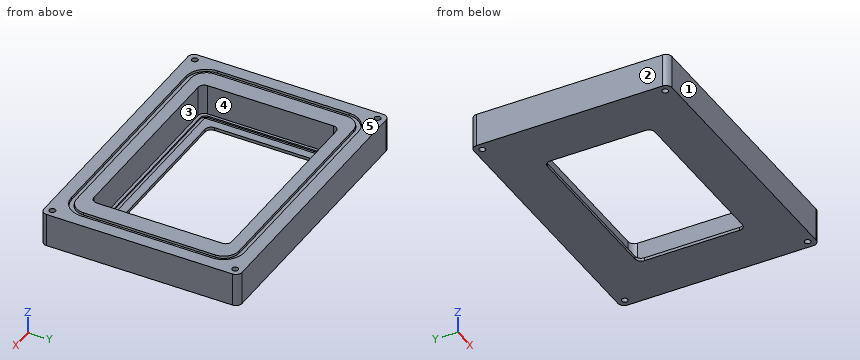
Autodesk Fusion 360 part; units mm, degrees
sketch "Sketch1" plane through (0, 0, 0) normal (0, 0, 1) x (1, 0, 0)
  line L0 (86, -65) -> (-86, -65)
  line L1 (-90, -61) -> (-90, 61)
  line L2 (-86, 65) -> (86, 65)
  line L3 (90, 61) -> (90, -61)
  line L4 (90, -65) -> (-90, 65) construction
  line L5 (-90, -65) -> (90, 65) construction
  arc A0 (-86, 65) -> (-90, 61) centre (-86, 61) ccw
  arc A1 (90, 61) -> (86, 65) centre (86, 61) ccw
  arc A2 (86, -65) -> (90, -61) centre (86, -61) ccw
  arc A3 (-90, -61) -> (-86, -65) centre (-86, -61) ccw
  circle A4 centre (-85, 60) radius 2
  line L6 (0, 65) -> (0, -65) construction
  line L7 (90, 0) -> (-90, 0) construction
  circle A5 centre (85, 60) radius 2
  circle A6 centre (85, -60) radius 2
  circle A7 centre (-85, -60) radius 2
  dimension "d1" = 180
  dimension "d2" = 130
  dimension "d26" = 4
  dimension "d27" = 4
  dimension "d28" = 4
  dimension "d29" = 4
  dimension "d30" = 4
  dimension "d31" = 5
  dimension "d32" = 5
extrude "Extrude1" add sketch "Sketch1" along normal blind 22
sketch "Sketch2" plane through (0, 0, 22) normal (0, 0, 1) x (-1, 0, 0)
  line L0 (-86, -65) -> (86, -65)
  line L1 (90, -61) -> (90, 61)
  line L2 (86, 65) -> (-86, 65)
  line L3 (-90, 61) -> (-90, -61)
  line L4 (-62.2, 45.25) -> (62.2, 45.25)
  line L5 (66.2, 41.25) -> (66.2, -41.25)
  line L6 (62.2, -45.25) -> (-62.2, -45.25)
  line L7 (-66.2, -41.25) -> (-66.2, 41.25)
  line L8 (-66.2, 45.25) -> (66.2, -45.25) construction
  line L9 (66.2, 45.25) -> (-66.2, -45.25) construction
  arc A0 (86, -65) -> (90, -61) centre (86, -61) ccw
  arc A1 (90, 61) -> (86, 65) centre (86, 61) ccw
  arc A2 (-86, 65) -> (-90, 61) centre (-86, 61) ccw
  arc A3 (-90, -61) -> (-86, -65) centre (-86, -61) ccw
  circle A4 centre (85, 60) radius 2
  circle A5 centre (-85, 60) radius 2
  circle A6 centre (-85, -60) radius 2
  circle A7 centre (85, -60) radius 2
  arc A8 (62.2, -45.25) -> (66.2, -41.25) centre (62.2, -41.25) ccw
  arc A9 (-66.2, -41.25) -> (-62.2, -45.25) centre (-62.2, -41.25) ccw
  arc A10 (66.2, 41.25) -> (62.2, 45.25) centre (62.2, 41.25) ccw
  arc A11 (-62.2, 45.25) -> (-66.2, 41.25) centre (-62.2, 41.25) ccw
  dimension "d5" = 132.4
  dimension "d6" = 90.5
  dimension "d52" = 4
  dimension "d53" = 4
  dimension "d54" = 4
  dimension "d55" = 4
extrude "Extrude2" cut sketch "Sketch2" against normal blind 20 contours L4 L5 L6 L7 A8 A9 A10 A11
sketch "Sketch3" plane through (0, 0, 22) normal (0, 0, 1) x (-1, 0, 0)
  line L0 (66.2, 41.25) -> (66.2, -41.25)
  line L1 (62.2, -45.25) -> (-62.2, -45.25)
  line L2 (-66.2, -41.25) -> (-66.2, 41.25)
  line L3 (-62.2, 45.25) -> (62.2, 45.25)
  line L4 (-86, -65) -> (86, -65)
  line L5 (90, -61) -> (90, 61)
  line L6 (86, 65) -> (-86, 65)
  line L7 (-90, 61) -> (-90, -61)
  line L8 (-79.9494, 54.9494) -> (79.9494, 54.9494) construction
  line L9 (79.9494, 54.9494) -> (79.9494, -54.9494) construction
  line L10 (79.9494, -54.9494) -> (-79.9494, -54.9494) construction
  line L11 (-79.9494, -54.9494) -> (-79.9494, 54.9494) construction
  line L12 (-79.9494, 54.9494) -> (79.9494, -54.9494) construction
  line L13 (79.9494, 54.9494) -> (-79.9494, -54.9494) construction
  line L14 (78.5149, 43.2459) -> (78.5149, -43.2459)
  line L15 (68.2459, -53.5149) -> (-68.2459, -53.5149)
  line L16 (-78.5149, -43.2459) -> (-78.5149, 43.2459)
  line L17 (-69.5341, 47.3937) -> (78.5149, -53.5149) construction
  line L18 (70.6619, 45.6619) -> (-70.6619, -45.6619) construction
  line L19 (-68.2459, 56.3839) -> (68.2459, 56.3839)
  line L20 (81.3839, 43.2459) -> (81.3839, -43.2459)
  line L21 (68.2459, -56.3839) -> (-68.2459, -56.3839)
  line L22 (-81.3839, -43.2459) -> (-81.3839, 43.2459)
  line L23 (-72.429, 50.1798) -> (81.3839, -56.3839) construction
  line L24 (73.5309, 48.5309) -> (-73.5309, -48.5309) construction
  arc A0 (68.2459, -53.5149) -> (78.5149, -43.2459) centre (68.2459, -43.2459) ccw
  arc A1 (68.2459, -56.3839) -> (81.3839, -43.2459) centre (68.2459, -43.2459) ccw
  line L25 (0, -65) -> (0, 65) construction
  line L26 (-90, 0) -> (90, 0) construction
  arc A2 (-78.5149, -43.2459) -> (-68.2459, -53.5149) centre (-68.2459, -43.2459) ccw
  arc A3 (-81.3839, -43.2459) -> (-68.2459, -56.3839) centre (-68.2459, -43.2459) ccw
  arc A4 (-68.2459, 53.5149) -> (-78.5149, 43.2459) centre (-68.2459, 43.2459) ccw
  arc A5 (-68.2459, 56.3839) -> (-81.3839, 43.2459) centre (-68.2459, 43.2459) ccw
  arc A6 (78.5149, 43.2459) -> (68.2459, 53.5149) centre (68.2459, 43.2459) ccw
  arc A7 (81.3839, 43.2459) -> (68.2459, 56.3839) centre (68.2459, 43.2459) ccw
  line L27 (-68.2459, 53.5149) -> (68.2459, 53.5149)
  arc A8 (86, -65) -> (90, -61) centre (86, -61) ccw
  arc A9 (90, 61) -> (86, 65) centre (86, 61) ccw
  arc A10 (-86, 65) -> (-90, 61) centre (-86, 61) ccw
  arc A11 (-90, -61) -> (-86, -65) centre (-86, -61) ccw
  circle A12 centre (85, 60) radius 2
  circle A13 centre (-85, 60) radius 2
  circle A14 centre (-85, -60) radius 2
  circle A15 centre (85, -60) radius 2
  arc A16 (66.2, 41.25) -> (62.2, 45.25) centre (62.2, 41.25) ccw
  arc A17 (62.2, -45.25) -> (66.2, -41.25) centre (62.2, -41.25) ccw
  arc A18 (-66.2, -41.25) -> (-62.2, -45.25) centre (-62.2, -41.25) ccw
  arc A19 (-62.2, 45.25) -> (-66.2, 41.25) centre (-62.2, 41.25) ccw
  dimension "d9" = 159.8988
  dimension "d15" = 109.8988
  dimension "d16" = 1.4345
  dimension "d17" = 1.4345
  dimension "d18" = 1.4345
  dimension "d19" = 1.4345
  dimension "d20" = 10.269
  dimension "d21" = 13.138
extrude "Extrude3" cut sketch "Sketch3" against normal blind 1.424 contours L19 L20 L21 L22 A1 A3 A5 A7
draft "Draft1" angle 10 neutral plane through (0, 0, 20.576) pull (0, 0, 1) 16 faces at (-78.5149, -14.4153, 21.5253) (-70.6669, 53.2254, 21.0507) (-22.7486, 53.5149, 21.5253) (74.2025, 51.6108, 21.0507) (78.5149, 14.4153, 21.0507) (71.6046, -52.9501, 21.5253) (22.7486, -53.5149, 21.5253) (-70.6669, -53.2254, 21.0507) (-81.3839, -14.4153, 21.5253) (-68.871, -56.369, 21.0507) (22.7486, -56.3839, 21.0507) (77.7543, -52.3122, 21.0507) (81.3839, 14.4153, 21.5253) (77.3122, 52.7543, 21.0507) (-22.7486, 56.3839, 21.0507) (-73.1288, 55.4428, 21.0507)
sketch "Sketch4" plane through (0, 0, 2) normal (0, 0, 1) x (-1, 0, 0)
  line L0 (-62.2, -45.25) -> (62.2, -45.25)
  line L1 (66.2, -41.25) -> (66.2, 41.25)
  line L2 (62.2, 45.25) -> (-62.2, 45.25)
  line L3 (-66.2, 41.25) -> (-66.2, -41.25)
  line L4 (-52.2, 35.25) -> (52.2, 35.25)
  line L5 (56.2, 31.25) -> (56.2, -31.25)
  line L6 (52.2, -35.25) -> (-52.2, -35.25)
  line L7 (-56.2, -31.25) -> (-56.2, 31.25)
  line L8 (-56.2, 35.25) -> (56.2, -35.25) construction
  line L9 (56.2, 35.25) -> (-56.2, -35.25) construction
  arc A0 (66.2, 41.25) -> (62.2, 45.25) centre (62.2, 41.25) ccw
  arc A1 (-62.2, 45.25) -> (-66.2, 41.25) centre (-62.2, 41.25) ccw
  arc A2 (-66.2, -41.25) -> (-62.2, -45.25) centre (-62.2, -41.25) ccw
  arc A3 (62.2, -45.25) -> (66.2, -41.25) centre (62.2, -41.25) ccw
  arc A4 (52.2, -35.25) -> (56.2, -31.25) centre (52.2, -31.25) ccw
  arc A5 (-56.2, -31.25) -> (-52.2, -35.25) centre (-52.2, -31.25) ccw
  arc A6 (-52.2, 35.25) -> (-56.2, 31.25) centre (-52.2, 31.25) ccw
  arc A7 (56.2, 31.25) -> (52.2, 35.25) centre (52.2, 31.25) ccw
  dimension "d35" = 10
  dimension "d36" = 10
  dimension "d71" = 4
  dimension "d72" = 4
  dimension "d73" = 4
  dimension "d74" = 4
extrude "Extrude4" cut sketch "Sketch4" against normal blind 5 contours L4 L5 L6 L7 A4 A5 A6 A7
sketch "Sketch6" plane through (0, 0, 2) normal (0, 0, 1) x (-1, 0, 0)
  line L0 (56.2, 31.25) -> (56.2, -31.25)
  line L1 (52.2, -35.25) -> (-52.2, -35.25)
  line L2 (-56.2, -31.25) -> (-56.2, 31.25)
  line L3 (-52.2, 35.25) -> (52.2, 35.25)
  arc A0 (66.2, 41.25) -> (62.2, 45.25) centre (62.2, 41.25) ccw
  line L4 (62.2, 45.25) -> (-62.2, 45.25)
  arc A1 (-62.2, 45.25) -> (-66.2, 41.25) centre (-62.2, 41.25) ccw
  line L5 (-66.2, 41.25) -> (-66.2, -41.25)
  arc A2 (-66.2, -41.25) -> (-62.2, -45.25) centre (-62.2, -41.25) ccw
  line L6 (-62.2, -45.25) -> (62.2, -45.25)
  arc A3 (62.2, -45.25) -> (66.2, -41.25) centre (62.2, -41.25) ccw
  line L7 (66.2, -41.25) -> (66.2, 41.25)
  arc A4 (60.9079, -41.3399) -> (62.4799, -39.7679) centre (60.9079, -39.7679) ccw construction
  arc A5 (-62.4799, -39.7399) -> (-60.9079, -41.3119) centre (-60.9079, -39.7399) ccw construction
  line L8 (-48.9575, -41.8399) -> (48.9575, -41.8399) construction
  line L9 (48.9575, 41.8399) -> (-48.9575, 41.8399) construction
  line L10 (-62.9799, 29.7119) -> (-62.9799, 27.8175) construction
  line L11 (48.9575, -41.8399) -> (50.8519, -41.8399) construction
  line L12 (62.4799, 30.3078) -> (62.4799, 39.7679) construction
  arc A6 (-60.88, 42.74) -> (-63.88, 39.74) centre (-60.88, 39.74) ccw construction
  line L13 (63.88, 39.74) -> (63.88, -39.74) construction
  arc A7 (63.88, 39.74) -> (60.88, 42.74) centre (60.88, 39.74) ccw construction
  line L14 (-62.9799, -29.7119) -> (-62.4799, -30.3078) construction
  line L15 (51.4478, 41.3399) -> (50.8519, 41.8399) construction
  arc A8 (60.88, -42.74) -> (63.88, -39.74) centre (60.88, -39.74) ccw construction
  line L16 (-48.9575, 41.8399) -> (-50.8519, 41.8399) construction
  line L17 (-60.88, 42.74) -> (60.88, 42.74) construction
  line L18 (-62.9799, -27.8175) -> (-62.9799, -29.7119) construction
  line L19 (60.88, -42.74) -> (-60.88, -42.74) construction
  line L20 (62.9799, 29.7119) -> (62.4799, 30.3078) construction
  line L21 (-50.8519, 41.8399) -> (-51.4811, 41.3119) construction
  line L22 (62.4799, -39.7679) -> (62.4799, -30.3078) construction
  line L23 (-50.8519, -41.8399) -> (-48.9575, -41.8399) construction
  line L24 (60.9079, 41.3399) -> (51.4478, 41.3399) construction
  line L25 (50.8519, 41.8399) -> (48.9575, 41.8399) construction
  line L26 (62.9799, 27.8175) -> (62.9799, 29.7119) construction
  line L27 (51.4478, -41.3399) -> (60.9079, -41.3399) construction
  line L28 (62.9799, -27.8175) -> (62.9799, 27.8175) construction
  line L29 (-63.88, -39.74) -> (-63.88, 39.74) construction
  line L30 (50.8519, -41.8399) -> (51.4478, -41.3399) construction
  line L31 (62.9799, -29.7119) -> (62.9799, -27.8175) construction
  arc A9 (-63.88, -39.74) -> (-60.88, -42.74) centre (-60.88, -39.74) ccw construction
  arc A10 (62.4799, 39.7679) -> (60.9079, 41.3399) centre (60.9079, 39.7679) ccw construction
  line L32 (62.4799, -30.3078) -> (62.9799, -29.7119) construction
  line L33 (-62.4799, 30.3078) -> (-62.9799, 29.7119) construction
  line L34 (-60.9079, -41.3119) -> (-51.4811, -41.3119) construction
  arc A11 (-60.9079, 41.3119) -> (-62.4799, 39.7399) centre (-60.9079, 39.7399) ccw construction
  line L35 (-51.4811, -41.3119) -> (-50.8519, -41.8399) construction
  line L36 (-51.4811, 41.3119) -> (-60.9079, 41.3119) construction
  line L37 (-62.4799, 39.7399) -> (-62.4799, 30.3078) construction
  line L38 (-62.4799, -30.3078) -> (-62.4799, -39.7399) construction
  line L39 (-62.9799, 27.8175) -> (-62.9799, -27.8175) construction
  line L40 (0, -45.25) -> (0, 45.25) construction
  line L41 (-66.2, 0) -> (66.2, 0) construction
  line L42 (-60.85, 43.25) -> (60.85, 43.25)
  line L43 (64.35, 39.75) -> (64.35, -39.75)
  line L44 (60.85, -43.25) -> (-60.85, -43.25)
  line L45 (-64.35, -39.75) -> (-64.35, 39.75)
  line L46 (-64.35, 43.25) -> (64.35, -43.25) construction
  line L47 (64.35, 43.25) -> (-64.35, -43.25) construction
  arc A12 (60.85, -43.25) -> (64.35, -39.75) centre (60.85, -39.75) ccw
  arc A13 (-64.35, -39.75) -> (-60.85, -43.25) centre (-60.85, -39.75) ccw
  arc A14 (-60.85, 43.25) -> (-64.35, 39.75) centre (-60.85, 39.75) ccw
  arc A15 (64.35, 39.75) -> (60.85, 43.25) centre (60.85, 39.75) ccw
  line L48 (-60.85, 40.75) -> (60.85, 40.75)
  line L49 (61.85, 39.75) -> (61.85, -39.75)
  line L50 (60.85, -40.75) -> (-60.85, -40.75)
  line L51 (-61.85, -39.75) -> (-61.85, 39.75)
  line L52 (-61.85, 40.75) -> (61.85, -40.75) construction
  line L53 (61.85, 40.75) -> (-61.85, -40.75) construction
  arc A16 (-61.85, -39.75) -> (-60.85, -40.75) centre (-60.85, -39.75) ccw
  arc A17 (60.85, -40.75) -> (61.85, -39.75) centre (60.85, -39.75) ccw
  arc A18 (61.85, 39.75) -> (60.85, 40.75) centre (60.85, 39.75) ccw
  arc A19 (-60.85, 40.75) -> (-61.85, 39.75) centre (-60.85, 39.75) ccw
  arc A20 (52.2, -35.25) -> (56.2, -31.25) centre (52.2, -31.25) ccw
  arc A21 (-56.2, -31.25) -> (-52.2, -35.25) centre (-52.2, -31.25) ccw
  arc A22 (-52.2, 35.25) -> (-56.2, 31.25) centre (-52.2, 31.25) ccw
  arc A23 (56.2, 31.25) -> (52.2, 35.25) centre (52.2, 31.25) ccw
  dimension "d56" = 128.7
  dimension "d57" = 86.5
  dimension "d58" = 3.5
  dimension "d59" = 3.5
  dimension "d60" = 3.5
  dimension "d61" = 3.5
  dimension "d63" = 2.5
  dimension "d64" = 2.5
  dimension "d65" = 1
  dimension "d66" = 1
  dimension "d67" = 1
  dimension "d68" = 1
extrude "Extrude6" cut sketch "Sketch6" against normal blind 1 contours L42 L43 L44 L45 A12 A13 A14 A15
equation "d9 = ( ORingPerimeter - 100 mm ) / 4 + 50 mm"
equation "ORingDiameter = 1.78 mm"
equation "ORingInnerDiameter = 170 mm"
equation "ORingPerimeter = 2 * 3.1412 * ( ( ORingInnerDiameter / 2 ) + ORingDiameter / 2 )"
equation "PanelWidth = 80 mm"
equation "PanelLength = 115 mm"
equation "d15 = ( ORingPerimeter - 100 mm ) / 4"
equation "d16 = ( ( ORingDiameter * 1.05 ) / 2 ) + 0.5 mm"
equation "d17 = ( ( ORingDiameter * 1.05 ) / 2 ) + 0.5 mm"
equation "d18 = ( ( ORingDiameter * 1.05 ) / 2 ) + 0.5 mm"
equation "d19 = ( ( ORingDiameter * 1.05 ) / 2 ) + 0.5 mm"
equation "d20 = ( ORingDiameter ) * 6 + ORingDiameter * 0.05 - 0.5 mm"
equation "d21 = ( ORingDiameter ) * 6 + ( ORingDiameter * 1.1 ) + 0.5 mm"
equation "d22 = -ORingDiameter * 0.8"
equation "ORing2Diameter = 2 mm"
equation "ORing2InnerDiameter = 126 mm"
equation "ORing2Perimeter = 2 * 3.1412 * ( ( ORing2InnerDiameter / 2 ) + ORing2Diameter / 2 )"
Read the model definition and answer for the solid it produces. Units are mm, in the model's axes. Face numbers are marked on the shaded views. A direction names the side the tool comes from. Give positions to 0.01 mm unless a question says otherwise; leave off trailing zeros. Write each loop counter-clockwise with the first axis right and the second up, starting at its lowest first coordinate (ties: lowest second). Pieces come first, ordered by that corner, then holes. Notation, with made-up numbers: (79, 19.5) - (91, 19.5) arc R22 cw to (91, 57.5) - close; hole circle Ø8 at (74, -17.5). An arc over 180 degrees is marked (long way). Write item = value, one per line. Start each with the question number.
Item 1: Find section B-B (z = 11.75). Give the vertices of the cut face in (x, y), then the cut area to 3 significant figures.
Item 2: Find section A-A (y = 27.5). Give the vertices of the cut face in (x, z), then the cut area to 3 significant figures.
Item 3: The mould has two halves that part along Y. Classify the marked faces 1, 2 and 3: +Y half, -Y half, draft (parallel to the pull), parting line (faces both ways), or undercut.
Item 4: Find the intervals of material crossed by probe 1 along Y at (x, z) = (85, 12.5); probe 2 along Y at (x, z) = (42.5, 1.25); probe 3 along X at (y, z) = (-36.5, 10), in increasing order. Write a range as [from, to].
Item 5: A tool of negligible diameter and unlimited length cuts with its end or side. For the marked faces 4 and 5, from which of +Z, -Z, +X, -X, +Y, -Y can it reach the whole face along a straight path? Write none if from no direction.
Item 6: This flat-tipped pin is pushed along its axis until it touches: P1, Ø12, axis at x = 26, y = -31.5, coming from the +Z side. Where does it stop, or does it pass through?
Response:
q1.outline = (-90, -61) arc R4 ccw to (-86, -65) - (86, -65) arc R4 ccw to (90, -61) - (90, 61) arc R4 ccw to (86, 65) - (-86, 65) arc R4 ccw to (-90, 61) - close; hole circle Ø4 at (-85, -60); hole circle Ø4 at (-85, 60); hole (-66.2, -41.25) arc R4 ccw to (-62.2, -45.25) - (62.2, -45.25) arc R4 ccw to (66.2, -41.25) - (66.2, 41.25) arc R4 ccw to (62.2, 45.25) - (-62.2, 45.25) arc R4 ccw to (-66.2, 41.25) - close; hole circle Ø4 at (85, -60); hole circle Ø4 at (85, 60)
q1.area = 11,400 mm²
q2.outline = (-90, 0) - (-56.2, 0) - (-56.2, 2) - (-61.85, 2) - (-61.85, 1) - (-64.35, 1) - (-64.35, 2) - (-66.2, 2) - (-66.2, 22) - (-78.26, 22) - (-78.51, 20.58) - (-81.38, 20.58) - (-81.63, 22) - (-90, 22) - close; (56.2, 0) - (90, 0) - (90, 22) - (81.63, 22) - (81.38, 20.58) - (78.51, 20.58) - (78.26, 22) - (66.2, 22) - (66.2, 2) - (64.35, 2) - (64.35, 1) - (61.85, 1) - (61.85, 2) - (56.2, 2) - close
q2.area = 1,070 mm²
q3.face_1 = -Y half
q3.face_2 = draft
q3.face_3 = undercut
q4.probe_1 = [-65, -62], [-58, 58], [62, 65]
q4.probe_2 = [-65, -43.25], [-40.75, -35.25], [35.25, 40.75], [43.25, 65]
q4.probe_3 = [-90, -66.2], [66.2, 90]
q5.face_4 = +Z
q5.face_5 = +Z, +X, -X, +Y, -Y
q6.P1 = 2
